Geometry: final body of the model. Coordinates: model frame, mm. A direction names the side the tool comes from. Coordinates: 2 decimals unless noted, no trailing zeros. Write each loop counter-clockwise with the first axis right and the second up, starting at its lowest first coordinate (ties: lowest second). Pieces come first, ordered by that corner, then holes.
from build123d import *

# Parameters (mm, degrees)
SKETCH1_R           = 1.75
BOSS_EXTRUDE1_DEPTH = 3


with BuildPart() as part:
    # Sketch1 → Boss-Extrude1 (new body)
    with BuildSketch(Plane.XY):
        with BuildLine():
            Line((-16.85, 4), (16.85, 4))
            ThreePointArc((16.85, 4), (20.85, 0), (16.85, -4))
            Line((16.85, -4), (16.85, -7))
            Line((16.85, -7), (7.15, -7))
            Line((7.15, -7), (7.15, -4))
            Line((7.15, -4), (-7.15, -4))
            Line((-7.15, -4), (-7.15, -7))
            Line((-7.15, -7), (-16.85, -7))
            Line((-16.85, -7), (-16.85, -4))
            ThreePointArc((-16.85, -4), (-20.85, 0), (-16.85, 4))
        make_face()
        with Locations((-16.85, 0)):
            Circle(SKETCH1_R, mode=Mode.SUBTRACT)
        with Locations((-8.425, 0)):
            Circle(SKETCH1_R, mode=Mode.SUBTRACT)
        Circle(SKETCH1_R, mode=Mode.SUBTRACT)
        with Locations((8.425, 0)):
            Circle(SKETCH1_R, mode=Mode.SUBTRACT)
        with Locations((16.85, 0)):
            Circle(SKETCH1_R, mode=Mode.SUBTRACT)
    extrude(amount=BOSS_EXTRUDE1_DEPTH)


solid = part.part
Item 1: Section B-B, the plane y = 0. Output: boundary loops of the cut face in (x, z) (3 decimals), plus the area to 3 significant figures.
Derived:
outline: (-20.85, 0) - (-18.6, 0) - (-18.6, 3) - (-20.85, 3) - close; (-15.1, 0) - (-10.175, 0) - (-10.175, 3) - (-15.1, 3) - close; (-6.675, 0) - (-1.75, 0) - (-1.75, 3) - (-6.675, 3) - close; (1.75, 0) - (6.675, 0) - (6.675, 3) - (1.75, 3) - close; (10.175, 0) - (15.1, 0) - (15.1, 3) - (10.175, 3) - close; (18.6, 0) - (20.85, 0) - (20.85, 3) - (18.6, 3) - close
area: 72.6 mm2
Item 2: Section A-A, the plane x = 0. Output: boundary loops of the cut face in (y, z).
Derived:
outline: (-4, 0) - (-1.75, 0) - (-1.75, 3) - (-4, 3) - close; (1.75, 0) - (4, 0) - (4, 3) - (1.75, 3) - close
Item 3: Set-up query: faces 1 (the cylindrical face through (1.617, -0.67, 1.479)), 2 (the flat face through (-12, -7, 1)), 3 (the flat face through (-16.85, -6, 1)), 4 (the flat face through (7.15, -6, 1)), 5 (the flat face through (16.85, -5, 1)). Return all of +Z, -Z, +X, -X, +Y, -Y with unobstructed straight access to the full face (end or side cutting, diameter ignored); none if empty.
Derived:
face 1: +Z, -Z
face 2: +Z, -Z, +X, -X, -Y
face 3: +Z, -Z, -X, -Y
face 4: +Z, -Z, -Y
face 5: +Z, -Z, +X, -Y
Item 4: Section D-D, the plane z = 1.4. Output: boundary loops of the cut face in (x, y) (3 decimals), plus the area to 3 significant figures.
Derived:
outline: (-16.85, -7) - (-7.15, -7) - (-7.15, -4) - (7.15, -4) - (7.15, -7) - (16.85, -7) - (16.85, -4) arc R4 ccw to (16.85, 4) - (-16.85, 4) arc R4 ccw to (-16.85, -4) - close; hole circle Ø3.5 at (-16.85, 0); hole circle Ø3.5 at (-8.425, 0); hole circle Ø3.5 at (0, 0); hole circle Ø3.5 at (8.425, 0); hole circle Ø3.5 at (16.85, 0)
area: 330 mm2
Item 5: Section C-C, the plane y = -4.5. Output: boundary loops of the cut face in (x, z), plus the area to 3 significant figures.
Derived:
outline: (-16.85, 0) - (-7.15, 0) - (-7.15, 3) - (-16.85, 3) - close; (7.15, 0) - (16.85, 0) - (16.85, 3) - (7.15, 3) - close
area: 58.2 mm2
Item 6: Pull-direction query (Y, two-part tool) for faces 6 (the flat face through (12, -7, 1)), 7 (the cylindrical face through (-10.173, 0.077, 1.479)), 8 (the flat face through (-7.15, -5, 1)); classes: released by +Y, released by -Y, zero draft, split by the parting line, or undercut.
Derived:
face 6: released by -Y
face 7: undercut
face 8: zero draft
Item 7: Pin query (flat end, axial travel): pin 1 (1.5 mm diameter, centred on y = -5.5, z = 2, fed in from +X); pin 2 (1.5 mm diameter, centred on x = 5.5, z = 1.5, fed in from -Y); pin 3 (3 mm diameter, centred on x = -8.425, y = 0, fed in from -Z). Return the tip coordinate at first contact, or that it passes through.
Derived:
pin 1: stops at x = 16.85
pin 2: stops at y = -4
pin 3: passes through
Item 8: Material intervals for probe 1 along X at (y, z) = (-5.5, 0.25); probe 2 along Y at (x, z) = (17, 1.1); probe 3 along X at (y, z) = (0.25, 0.6), sorted ascending.
Derived:
probe 1: x = -16.85 to -7.15, 7.15 to 16.85
probe 2: y = -4 to -1.74, 1.74 to 4
probe 3: x = -20.84 to -18.58, -15.12 to -10.16, -6.69 to -1.73, 1.73 to 6.69, 10.16 to 15.12, 18.58 to 20.84
